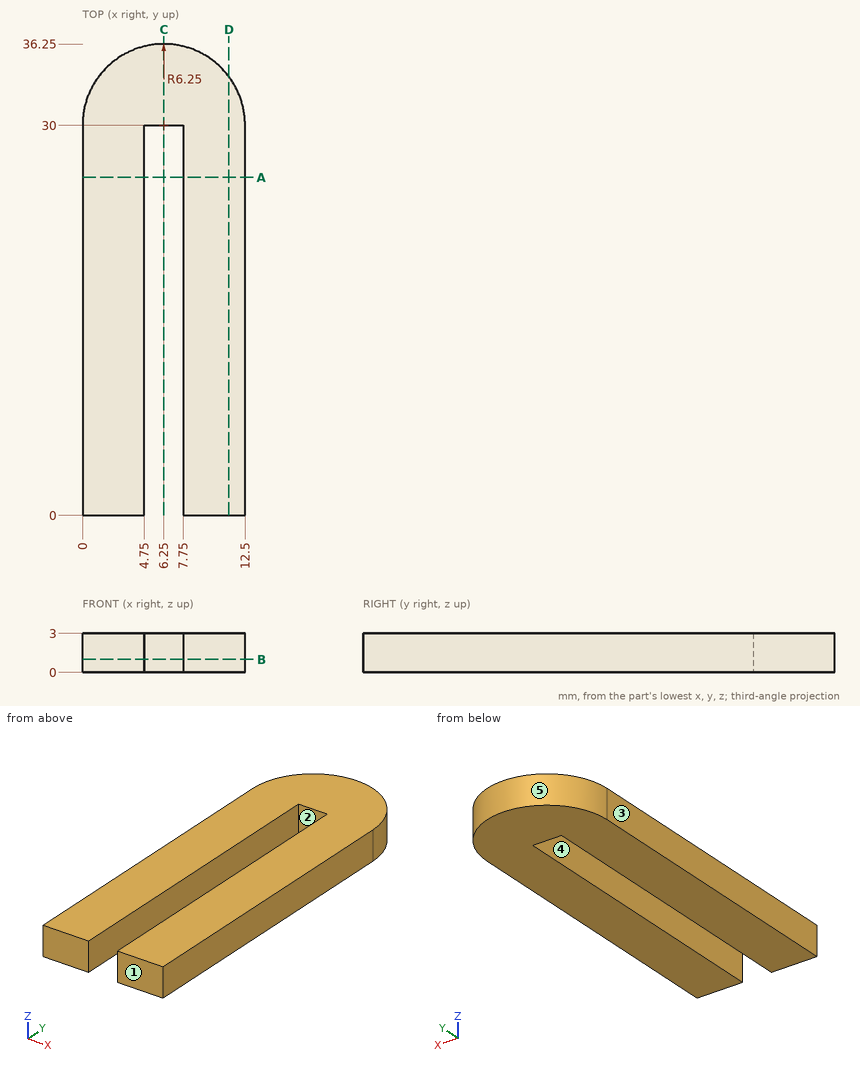
Design review of the part shown in the three views and the two pictorial views. Dimensions are in mm from the part's minimum x, y and z. A direction names the side the tool comes from. Give positions to 0.01 mm unless a question says otherwise; leave off trailing zeros. Loops run counter-clockwise (first coordinate to the right, second up) from the corner with the lowest first, then second, coordinate; pieces in that order, holes last. Notation, with made-up numbers: (52, -13.5) -> (89, -13.5) arc R15 ccw to (89, -3.5) -> close; hole circle Ø2 at (80, 77.5). An arc over 180 degrees is marked (long way). Put each result on its own line as item: value. Start each with the question number.
1. Wall thickness on probe 1 along X at (y, z) = (26, 2.3); probe 2 along Y at (x, z) = (12, 1); probe 3 along X at (y, z) = (30.5, 2.25): over which ranges is each line inside the solid? List them lowest first.
2. For the marked faces 4 and 5, list the 3-axis set-ups (+Z, -Z, +X, -X, +Y, -Y) from which the entire face can be reached by the end or side of a thin tool; tool diameter is ignored.
3. We need section D-D on x = 11.25. State the section outline as (y, z) points, then the cut area to 3 significant figures.
4. Mouldability with a two-part tool opening along X and no side actions: class the marked faces 1, 2 and 3 as released by +X, released by -X, zero draft, split by the parting line, or undercut.
5. We need section A-A on y = 26. State the section outline as (x, z) points, then the cut area to 3 significant figures.
6. We need section C-C on x = 6.25. State the section outline as (y, z) points, then the cut area to 4 significant figures.
7. Clearance check with a flat-ended pin moving along its axis: P1, Ø1.5, axis at x = 6.5, y = 24, coming from the -Z side. State where the tip first meets the part, or that it passes through.
8. We need section B-B on z = 1. State the section outline as (x, y) points, then the cut area to 3 significant figures.
Determined:
1. probe 1: 0 to 4.75, 7.75 to 12.5
1. probe 2: 0 to 32.45
1. probe 3: 0.02 to 12.48
2. face 4: +Z, -Z, -Y
2. face 5: +Z, -Z, +Y
3. outline: (0, 0) -> (33.75, 0) -> (33.75, 3) -> (0, 3) -> close
3. area: 101 mm^2
4. face 1: zero draft
4. face 2: undercut
4. face 3: released by -X
5. outline: (0, 0) -> (4.75, 0) -> (4.75, 3) -> (0, 3) -> close; (7.75, 0) -> (12.5, 0) -> (12.5, 3) -> (7.75, 3) -> close
5. area: 28.5 mm^2
6. outline: (30, 0) -> (36.25, 0) -> (36.25, 3) -> (30, 3) -> close
6. area: 18.75 mm^2
7. P1: through
8. outline: (0, 0) -> (4.75, 0) -> (4.75, 30) -> (7.75, 30) -> (7.75, 0) -> (12.5, 0) -> (12.5, 30) arc R6.25 ccw to (0, 30) -> close
8. area: 346 mm^2
